Read the model definition and answer for the solid it produces. Units are mm, in the model's axes. Face numbers are marked on the shaded views. Give positions to 0.01 mm unless a question says otherwise; leave off trailing zeros. Use a Markdown table: item, result. Add a question column.
1. For a pull along Z with two mould halves and no side action, classify the marked faces 1 and 2 as released by +Z, released by -Z, zero draft, split by the parting line, or undercut.
2. Flat-ended cylindrical pins translate along their axes: P1, Ø6, axis at x = 26.5, z = -2.5, coming from the -Y side; P2, Ø1, axis at x = -12, z = 15.5, coming from the -Y side; P3, Ø3, axis at x = -4.5, z = 46.5, coming from the -Y side. Find the tip coordinate at first contact, or state that the pin passes through.
3. Consider L1, parallel to X at y = -2, z = -7; L2, parallel to Y at x = 33.5, z = 22.5; L3, parallel to Z at x = 7.5, y = -4.25. Determine where each line is inside the solid, lowest interval first.
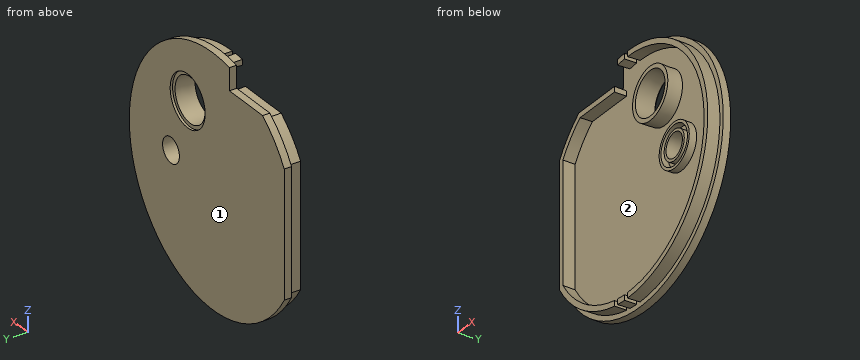
```python
from build123d import *

# Parameters (mm, degrees)
BOSS_EXTRUDE1_DEPTH           = 3
BOSS_EXTRUDE1_DRAFT           = -1
BOSS_EXTRUDE2_DEPTH           = 5
BOSS_EXTRUDE2_DRAFT           = -1
BOSS_EXTRUDE2_PROFILE_2_DEPTH = 5
BOSS_EXTRUDE2_PROFILE_2_DRAFT = -1
BOSS_EXTRUDE2_PROFILE_3_DEPTH = 5
BOSS_EXTRUDE2_PROFILE_3_DRAFT = -1
BOSS_EXTRUDE2_PROFILE_4_DEPTH = 5
BOSS_EXTRUDE2_PROFILE_4_DRAFT = -1
SKETCH3_R                     = 5
CUT_EXTRUDE1_DEPTH            = 3
CUT_EXTRUDE1_DRAFT            = 1
SKETCH3_R_2                   = 9
CUT_EXTRUDE1_PROFILE_2_DEPTH  = 3
CUT_EXTRUDE1_PROFILE_2_DRAFT  = 1
SKETCH4_R                     = 9
SKETCH4_R_2                   = 8
BOSS_EXTRUDE3_DEPTH           = 3
BOSS_EXTRUDE3_DRAFT           = -1
SKETCH4_3_R                   = 6
SKETCH4_3_R_2                 = 5
BOSS_EXTRUDE4_DEPTH           = 3
BOSS_EXTRUDE4_DRAFT           = -1
SKETCH6_R                     = 10.5
SKETCH6_R_2                   = 9
BOSS_EXTRUDE5_DEPTH           = 6
BOSS_EXTRUDE5_DRAFT           = -1
SKETCH7_R                     = 10.5
SKETCH7_R_2                   = 9
CUT_EXTRUDE2_DEPTH            = 1
CUT_EXTRUDE2_DRAFT            = 1


with BuildPart() as part:
    # Sketch1 → Boss-Extrude1 (with draft: the straight prism first)
    with BuildSketch(Plane(origin=(0, 0, 0), x_dir=(1, 0, 0), z_dir=(0, 1, 0))):
        with BuildLine():
            Line((-43, 25.514701644), (-43, -25.514701644))
            ThreePointArc((-43, -25.514701644), (-37.211637523, -33.396018219), (-30, -40))
            Line((-30, -40), (-10, -40))
            Line((-10, -40), (-10, -48.989794856))
            ThreePointArc((-10, -48.989794856), (45.716299059, 20.248950598), (-43, 25.514701644))
        make_face()
    extrude(amount=BOSS_EXTRUDE1_DEPTH)
    # Boss-Extrude1: the draft: its side faces are tilted about the plane it starts from
    boss_extrude1_sides = [part.faces().sort_by_distance(p)[0] for p in [
        (-43, 1.5, 0),
        (-37.211637523, 1.5, 33.396018219),
        (-20, 1.5, 40),
        (-10, 1.5, 44.494897428),
        (45.716299059, 1.5, -20.248950598),
    ]]
    draft(boss_extrude1_sides, Plane(origin=(0, 0, 0), x_dir=(1, 0, 0), z_dir=(0, 1, 0)), BOSS_EXTRUDE1_DRAFT)


with BuildPart() as boss_extrude2_tool:
    # Sketch2 → Boss-Extrude2 (with draft: the straight prism first)
    with BuildSketch(Plane.XZ):
        with BuildLine():
            Line((-40.978122, 24.995870006), (-40.978122, -24.995870006))
            ThreePointArc((-40.978122, -24.995870006), (-26.914721681, -39.744153744), (-8, -47.328638265))
            Line((-8, -47.328638265), (-8, -45.299006612))
            ThreePointArc((-8, -45.299006612), (-25.702922785, -38.149177715), (-38.978122, -24.427566505))
            Line((-38.978122, -24.427566505), (-38.978122, 24.427566505))
            ThreePointArc((-38.978122, 24.427566505), (-34.298477795, 30.653130687), (-28.635642127, 36))
            Line((-28.635642127, 36), (-8, 36))
            Line((-8, 36), (-8, 38))
            Line((-8, 38), (-29.325756597, 38))
            ThreePointArc((-29.325756597, 38), (-35.748226329, 32.032238672), (-40.978122, 24.995870006))
        make_face()
    extrude(amount=BOSS_EXTRUDE2_DEPTH)
    # Boss-Extrude2: the draft: its side faces are tilted about the plane it starts from
    boss_extrude2_sides = [boss_extrude2_tool.faces().sort_by_distance(p)[0] for p in [
        (-38.978122, -2.5, 0),
        (-34.298477795, -2.5, 30.653130687),
        (-18.317821063, -2.5, 36),
        (-8, -2.5, 37),
        (-18.662878299, -2.5, 38),
        (-35.748226329, -2.5, 32.032238672),
        (-40.978122, -2.5, 0),
        (-26.914721681, -2.5, -39.744153744),
        (-8, -2.5, -46.313822438),
        (-25.702922785, -2.5, -38.149177715),
    ]]
    draft(boss_extrude2_sides, Plane.XZ, BOSS_EXTRUDE2_DRAFT)


with BuildPart() as part_1:
    add(part.part)

    # Boss-Extrude2: add boss_extrude2_tool
    add(boss_extrude2_tool.part)


with BuildPart() as boss_extrude2_profile_2_tool:
    # Sketch2 → Boss-Extrude2 profile 2 (with draft: the straight prism first)
    with BuildSketch(Plane.XZ):
        with BuildLine():
            ThreePointArc((-6, 45.607017004), (-4.00381503, 45.825423786), (-2, 45.956501172))
            Line((-2, 45.956501172), (-2, 47.958315233))
            ThreePointArc((-2, 47.958315233), (-4.003501138, 47.832750064), (-6, 47.623523599))
            Line((-6, 47.623523599), (-6, 45.607017004))
        make_face()
    extrude(amount=BOSS_EXTRUDE2_PROFILE_2_DEPTH)
    # Boss-Extrude2 profile 2: the draft: its side faces are tilted about the plane it starts from
    boss_extrude2_profile_2_sides = [boss_extrude2_profile_2_tool.faces().sort_by_distance(p)[0] for p in [
        (-4.00381503, -2.5, 45.825423786),
        (-2, -2.5, 46.957408203),
        (-4.003501138, -2.5, 47.832750064),
        (-6, -2.5, 46.615270302),
    ]]
    draft(boss_extrude2_profile_2_sides, Plane.XZ, BOSS_EXTRUDE2_PROFILE_2_DRAFT)


with BuildPart() as part_2:
    add(part_1.part)

    # Boss-Extrude2 profile 2: add boss_extrude2_profile_2_tool
    add(boss_extrude2_profile_2_tool.part)


with BuildPart() as boss_extrude2_profile_3_tool:
    # Sketch2 → Boss-Extrude2 profile 3 (with draft: the straight prism first)
    with BuildSketch(Plane.XZ):
        with BuildLine():
            Line((-6, -45.607017004), (-6, -47.623523599))
            ThreePointArc((-6, -47.623523599), (-4.003501138, -47.832750064), (-2, -47.958315233))
            Line((-2, -47.958315233), (-2, -45.956501172))
            ThreePointArc((-2, -45.956501172), (-4.00381503, -45.825423786), (-6, -45.607017004))
        make_face()
    extrude(amount=BOSS_EXTRUDE2_PROFILE_3_DEPTH)
    # Boss-Extrude2 profile 3: the draft: its side faces are tilted about the plane it starts from
    boss_extrude2_profile_3_sides = [boss_extrude2_profile_3_tool.faces().sort_by_distance(p)[0] for p in [
        (-4.00381503, -2.5, -45.825423786),
        (-6, -2.5, -46.615270302),
        (-4.003501138, -2.5, -47.832750064),
        (-2, -2.5, -46.957408203),
    ]]
    draft(boss_extrude2_profile_3_sides, Plane.XZ, BOSS_EXTRUDE2_PROFILE_3_DRAFT)


with BuildPart() as part_3:
    add(part_2.part)

    # Boss-Extrude2 profile 3: add boss_extrude2_profile_3_tool
    add(boss_extrude2_profile_3_tool.part)


with BuildPart() as boss_extrude2_profile_4_tool:
    # Sketch2 → Boss-Extrude2 profile 4 (with draft: the straight prism first)
    with BuildSketch(Plane.XZ):
        with BuildLine():
            ThreePointArc((0, 46), (46, 0), (0, -46))
            Line((0, -46), (0, -48))
            ThreePointArc((0, -48), (48, 0), (0, 48))
            Line((0, 48), (0, 46))
        make_face()
    extrude(amount=BOSS_EXTRUDE2_PROFILE_4_DEPTH)
    # Boss-Extrude2 profile 4: the draft: its side faces are tilted about the plane it starts from
    boss_extrude2_profile_4_sides = [boss_extrude2_profile_4_tool.faces().sort_by_distance(p)[0] for p in [
        (0, -2.5, -47),
        (48, -2.5, 0),
        (0, -2.5, 47),
        (46, -2.5, 0),
    ]]
    draft(boss_extrude2_profile_4_sides, Plane.XZ, BOSS_EXTRUDE2_PROFILE_4_DRAFT)


with BuildPart() as part_4:
    add(part_3.part)

    # Boss-Extrude2 profile 4: add boss_extrude2_profile_4_tool
    add(boss_extrude2_profile_4_tool.part)


with BuildPart() as cut_extrude1_tool:
    # Sketch3 → Cut-Extrude1 (with draft: the straight prism first)
    with BuildSketch(Plane.XZ):
        with Locations((25, 0)):
            Circle(SKETCH3_R)
    extrude(amount=-CUT_EXTRUDE1_DEPTH)
    # Cut-Extrude1: the draft: its side faces are tilted about the plane it starts from
    cut_extrude1_sides = [cut_extrude1_tool.faces().sort_by_distance(p)[0] for p in [
        (20, 1.5, 0),
    ]]
    draft(cut_extrude1_sides, Plane.XZ, CUT_EXTRUDE1_DRAFT)


with BuildPart() as part_5:
    add(part_4.part)

    # Cut-Extrude1: cut by cut_extrude1_tool
    add(cut_extrude1_tool.part, mode=Mode.SUBTRACT)


with BuildPart() as cut_extrude1_profile_2_tool:
    # Sketch3 → Cut-Extrude1 profile 2 (with draft: the straight prism first)
    with BuildSketch(Plane.XZ):
        with Locations((15, 24)):
            Circle(SKETCH3_R_2)
    extrude(amount=-CUT_EXTRUDE1_PROFILE_2_DEPTH)
    # Cut-Extrude1 profile 2: the draft: its side faces are tilted about the plane it starts from
    cut_extrude1_profile_2_sides = [cut_extrude1_profile_2_tool.faces().sort_by_distance(p)[0] for p in [
        (6, 1.5, 24),
    ]]
    draft(cut_extrude1_profile_2_sides, Plane.XZ, CUT_EXTRUDE1_PROFILE_2_DRAFT)


with BuildPart() as part_6:
    add(part_5.part)

    # Cut-Extrude1 profile 2: cut by cut_extrude1_profile_2_tool
    add(cut_extrude1_profile_2_tool.part, mode=Mode.SUBTRACT)


with BuildPart() as boss_extrude3_tool:
    # Sketch4 → Boss-Extrude3 (with draft: the straight prism first)
    with BuildSketch(Plane.XZ):
        with Locations((25, 0)):
            Circle(SKETCH4_R)
        with Locations((25, 0)):
            Circle(SKETCH4_R_2, mode=Mode.SUBTRACT)
    extrude(amount=BOSS_EXTRUDE3_DEPTH)
    # Boss-Extrude3: the draft: its side faces are tilted about the plane it starts from
    boss_extrude3_sides = [boss_extrude3_tool.faces().sort_by_distance(p)[0] for p in [
        (16, -1.5, 0),
        (17, -1.5, 0),
    ]]
    draft(boss_extrude3_sides, Plane.XZ, BOSS_EXTRUDE3_DRAFT)


with BuildPart() as part_7:
    add(part_6.part)

    # Boss-Extrude3: add boss_extrude3_tool
    add(boss_extrude3_tool.part)


with BuildPart() as boss_extrude4_tool:
    # Sketch4<3> → Boss-Extrude4 (with draft: the straight prism first)
    with BuildSketch(Plane.XZ):
        with Locations((25, 0)):
            Circle(SKETCH4_3_R)
        with Locations((25, 0)):
            Circle(SKETCH4_3_R_2, mode=Mode.SUBTRACT)
    extrude(amount=BOSS_EXTRUDE4_DEPTH)
    # Boss-Extrude4: the draft: its side faces are tilted about the plane it starts from
    boss_extrude4_sides = [boss_extrude4_tool.faces().sort_by_distance(p)[0] for p in [
        (19, -1.5, 0),
        (20, -1.5, 0),
    ]]
    draft(boss_extrude4_sides, Plane.XZ, BOSS_EXTRUDE4_DRAFT)


with BuildPart() as part_8:
    add(part_7.part)

    # Boss-Extrude4: add boss_extrude4_tool
    add(boss_extrude4_tool.part)


with BuildPart() as boss_extrude5_tool:
    # Sketch6 → Boss-Extrude5 (with draft: the straight prism first)
    with BuildSketch(Plane.XZ):
        with Locations((15, 24)):
            Circle(SKETCH6_R)
        with Locations((15, 24)):
            Circle(SKETCH6_R_2, mode=Mode.SUBTRACT)
    extrude(amount=BOSS_EXTRUDE5_DEPTH)
    # Boss-Extrude5: the draft: its side faces are tilted about the plane it starts from
    boss_extrude5_sides = [boss_extrude5_tool.faces().sort_by_distance(p)[0] for p in [
        (4.5, -3, 24),
        (6, -3, 24),
    ]]
    draft(boss_extrude5_sides, Plane.XZ, BOSS_EXTRUDE5_DRAFT)


with BuildPart() as part_9:
    add(part_8.part)

    # Boss-Extrude5: add boss_extrude5_tool
    add(boss_extrude5_tool.part)


with BuildPart() as cut_extrude2_tool:
    # Sketch7 → Cut-Extrude2 (with draft: the straight prism first)
    with BuildSketch(Plane(origin=(0, 3, 0), x_dir=(1, 0, 0), z_dir=(0, 1, 0))):
        with Locations((15, -24)):
            Circle(SKETCH7_R)
        with Locations((15, -24)):
            Circle(SKETCH7_R_2, mode=Mode.SUBTRACT)
    extrude(amount=-CUT_EXTRUDE2_DEPTH)
    # Cut-Extrude2: the draft: its side faces are tilted about the plane it starts from
    cut_extrude2_sides = [cut_extrude2_tool.faces().sort_by_distance(p)[0] for p in [
        (4.5, 2.5, 24),
        (6, 2.5, 24),
    ]]
    draft(cut_extrude2_sides, Plane(origin=(0, 3, 0), x_dir=(1, 0, 0), z_dir=(0, 1, 0)), CUT_EXTRUDE2_DRAFT)


with BuildPart() as part_10:
    add(part_9.part)

    # Cut-Extrude2: cut by cut_extrude2_tool
    add(cut_extrude2_tool.part, mode=Mode.SUBTRACT)


solid = part_10.part
```
Output values:
| question | item | result |
|---|---|---|
| 1 | face 1 | zero draft |
| 1 | face 2 | undercut |
| 2 | P1 | y = -3 |
| 2 | P2 | y = 0 |
| 2 | P3 | y = -5 |
| 3 | L1 | -41.01 to -38.94, 19.29 to 21.2, 28.8 to 30.71, 45.43 to 47.52 |
| 3 | L2 | 0 to 3 |
| 3 | L3 | -47.49 to -45.31, 16.55 to 19.16, 28.84 to 31.45, 45.31 to 47.49 |
